```python
from build123d import *

# Parameters (mm, degrees)
F0_W     = 83.8454
F0_H     = 28.3464
F0_R     = 10.9982
F1_DEPTH = 3.5052
F2_R     = 12.7


with BuildPart() as f1:
    # F0 (on Front) → F1 (new body, symmetric)
    with BuildSketch(Plane.XZ):
        with Locations((4.0005, 0)):
            Rectangle(F0_W, F0_H)
        with BuildLine():
            ThreePointArc((-34.2646, 1.630949), (-30.899574, 2.874019), (-28.7528, 0))
            ThreePointArc((-28.7528, 0), (-30.899574, -2.874019), (-34.2646, -1.630949))
            ThreePointArc((-34.2646, -1.630949), (-34.7472, 0), (-34.2646, 1.630949))
        make_face(mode=Mode.SUBTRACT)
        with Locations((31.75, 0)):
            Circle(F0_R, mode=Mode.SUBTRACT)
        with BuildLine():
            Line((-34.2646, -1.630949), (-34.2646, 1.630949))
            ThreePointArc((-34.2646, 1.630949), (-34.7472, 0), (-34.2646, -1.630949))
        make_face()
    extrude(amount=F1_DEPTH, both=True)

    # F2
    f2_edges = [f1.edges().sort_by_distance(p)[0] for p in [
        (-37.9222, 0, 14.1732),
        (-37.9222, 0, -14.1732),
        (45.9232, 0, 14.1732),
        (45.9232, 0, -14.1732),
    ]]
    fillet(f2_edges, radius=F2_R)


solid = f1.part
```
For this review, take the finished solid that the model builds, in its own axes (mm). Coordinates: 2 decimals unless noted, no trailing zeros. Loops run counter-clockwise (first coordinate to the right, second up) from the corner with the lowest first, then second, coordinate; pieces in that order, holes last.
1. Mouldability with a two-part tool opening along X and no side actions: class faces 1 (the flat face through (-34.265, 0, 0)), 2 (the flat face through (45.923, 0, 0)), 3 (the flat face through (-6, 3.505, 0)) as +X half, -X half, draft (parallel to the pull), parting line (faces both ways), or undercut.
2. Add section C-C, the plane y = -1.5. Give the boundary of the cut face in (x, z).
3. Add section B-B, the plane z = 9. Give the boundary of the cut face in (x, y), then the cut area to 3 significant figures.
4. Add section A-A, the plane x = 31.75. Give the boundary of the cut face in (y, z).
5. For line 1 (Z direction, x = 31.75, y = -0.5); line 2 (Z direction, x = 24, y = 2.5); line 3 (X direction, y = 0.5, z = -7), list the stretches that pass through material, from the lowest coordinate up.
Result:
1. face 1: undercut
1. face 2: +X half
1. face 3: draft
2. outline: (-37.92, -1.47) arc R12.7 ccw to (-25.22, -14.17) - (33.22, -14.17) arc R12.7 ccw to (45.92, -1.47) - (45.92, 1.47) arc R12.7 ccw to (33.22, 14.17) - (-25.22, 14.17) arc R12.7 ccw to (-37.92, 1.47) - close; hole (-34.26, -1.63) arc R3 ccw (long way) to (-34.26, 1.63) - close; hole circle Ø22 at (31.75, 0)
3. outline: (-35.45, -3.51) - (25.43, -3.51) - (25.43, 3.51) - (-35.45, 3.51) - close; (38.07, -3.51) - (43.45, -3.51) - (43.45, 3.51) - (38.07, 3.51) - close
3. area: 465 mm2
4. outline: (-3.51, -14.17) - (3.51, -14.17) - (3.51, -11) - (-3.51, -11) - close; (-3.51, 11) - (3.51, 11) - (3.51, 14.17) - (-3.51, 14.17) - close
5. line 1: z = -14.17 to -11, 11 to 14.17
5. line 2: z = -14.17 to -7.8, 7.8 to 14.17
5. line 3: x = -36.66 to 23.27, 40.23 to 44.66
